Input: part model. Units: mm. Frame: model coordinates. A direction names the side the tool comes from. Round coordinates to 2 decimals unless told otherwise and drop trailing zeros. Loops run counter-clockwise (first coordinate to the right, second up) from the corner with the lowest first, then second, coordinate; pieces in that order, holes last.
1) Section C-C, the plane z = 272. Return loops of the section in (x, y), and give its area (3 significant figures).
2) First-contact query: pin 1 (5 mm diameter, centred on x = 432.5, z = 73.5, fed in from +Y); pin 2 (1.5 mm diameter, centred on y = 10, z = 263.5, fed in from -X); pin 3 (24 mm diameter, centred on x = -34, z = 3, fed in from +Y); pin 4 (12 mm diameter, centred on y = 4.5, z = 322.5, fed in from -X). Flat tips, straight axial feed; report the tip coordinate or a pass-through.
3) Access query for faces 5 (the face through (-5, 15, 0)), 6 (the face through (125, 15, 15)), 7 (the face through (-27, 45, 0)). Directions: +Z, -Z, +X, -X, +Y, -Y. A direction counts if a zero-diameter tool reaches every point of the face in a straight line with its end or side. Return the directions, or none.
4) Section A-A, the plane y = 13. Return loops of the section in (x, z), and give its area (3 significant figures).
5) Section B-B, the plane x = 766.5. Return loops of the section in (y, z).
6) Draft query along Y for faces 1 (the face through (697, 30, 240)), 2 (the face through (1285.01, 14.79, 568.91)), 3 (the face through (697, 0, 240)), 4 (the face through (-30, 30, 0)). Return one class per face: pulls with the +Y half, pulls with the -Y half, needs draft (parallel to the pull), parting line crosses it, or undercut.
7) Ray query, line 1 along Z through (x, y) = (300, 18.5); line 2 along Z through (x, y) = (-40, 40); line 3 along X through (y, z) = (-4.5, 0). Return the intervals inside material, ascending.
Autodesk Inventor part; units mm, degrees
ref_plane "Płaszczyzna konstrukcyjna1" through (0, 15, 0) normal (0, 1, 0) x (-1, 0, 0)
ref_plane "YZ Plane" through (0, 0, 0) normal (1, 0, 0) x (0, 1, 0)
ref_plane "XY Plane" through (0, 0, 0) normal (0, 0, 1) x (1, 0, 0)
sketch "Szkic1" plane through (0, 0, 0) normal (0, 1, 0) x (-1, 0, 0)
  line L0 (0, 15) -> (-300, 15)
  line L1 (-300, 15) -> (-300, -15)
  line L2 (-300, -15) -> (0, -15)
  line L3 (0, -15) -> (0, 15)
  line L4 (-300, 15) -> (-1278.6087, 580)
  line L5 (-1278.6087, 580) -> (-1291.5991, 557.5)
  line L6 (-300, -15) -> (-1291.5991, 557.5)
  point P0 (0, 0)
  point P1 (0, 0)
  dimension "d0" = 300
  dimension "d1" = 30
  dimension "d2" = 150
  dimension "d3" = 1130
extrude "Wyciągnięcie proste1" add sketch "Szkic1" along normal blind 30
sketch "Szkic2" plane through (0, 30, 0) normal (0, 1, 0) x (1, 0, 0)
  circle A0 centre (300, 0) radius 10
  line L0 (300, 15) -> (0, 15)
  point P0 (0, 0)
  dimension "d6" = 20
  dimension "d7" = 15
extrude "Wyciągnięcie proste2" cut sketch "Szkic2" against normal through all
sketch "Szkic3" plane through (0, 0, -15) normal (-1, 0, 0) x (0, 0, 1)
  point P0 (15, 0)
sketch "Szkic4" plane through (0, 0, -15) normal (-1, 0, 0) x (0, 0, 1)
  line L0 (0, 0) -> (30, 0)
  line L1 (30, 0) -> (30, 30)
  line L2 (0, 30) -> (30, 30)
  line L3 (0, 0) -> (0, 30)
  line L4 (30, 45) -> (0, 45)
  line L5 (0, 45) -> (0, -15)
  line L6 (0, -15) -> (30, -15)
  line L7 (30, -15) -> (30, 45)
  line L8 (30, 45) -> (0, -15) construction
  line L9 (0, 45) -> (30, -15) construction
  point P0 (15, 0)
  point P1 (15, 15)
  dimension "d10" = 30
  dimension "d11" = 60
  dimension "d12" = 0
  dimension "d13" = 15
extrude "Wyciągnięcie proste3" add sketch "Szkic4" along normal blind 5
sketch "Szkic5" plane through (-5, 0, -15) normal (-1, 0, 0) x (0, 0, 1)
  line L0 (0, -15) -> (30, -15)
  line L1 (30, -15) -> (30, 0)
  line L2 (30, 0) -> (0, 0)
  line L3 (0, 0) -> (0, -15)
  point P0 (15, 0)
  dimension "d16" = 30
  dimension "d17" = 15
extrude "Wyciągnięcie proste4" add sketch "Szkic5" along normal blind 50
ref_plane "Płaszczyzna konstrukcyjna1" through (0, 15, 0) normal (0, 1, 0) x (-1, 0, 0)
mirror "Odbicie lustrzane1" about plane through (0, 15, 0) normal (0, 1, 0) of "Wyciągnięcie proste4"
sketch "Szkic6" plane through (0, 45, 15) normal (0, 1, 0) x (1, 0, 0)
  circle A0 centre (-40, 15) radius 7.5
  line L0 (-55, 30) -> (-55, 0)
  line L1 (0, 0) -> (0, 30)
  point P0 (0, 15)
  point P1 (0, 15)
  dimension "d21" = 15
  dimension "d22" = 15
extrude "Wyciągnięcie proste5" cut sketch "Szkic6" against normal through all
properties part number "3" material "Złote"
Final values:
1. outline: (745.14, 0) - (797.1, 0) - (797.1, 30) - (745.14, 30) - close
1. area: 1,560 mm2
2. pin 1: stops at y = 30
2. pin 2: stops at x = 729.12
2. pin 3: stops at y = 45
2. pin 4: stops at x = 822.21
3. face 5: +Z, -Z, -X
3. face 6: +Z, -X, +Y, -Y
3. face 7: +Z, -Z, +X, -X, +Y
4. outline: (-5, -15) - (300, -15) - (1291.6, 557.5) - (1278.61, 580) - (300, 15) - (-5, 15) - close; hole circle Ø20 at (300, 0)
4. area: 38,400 mm2
5. outline: (0, 254.33) - (30, 254.33) - (30, 284.33) - (0, 284.33) - close
6. face 1: pulls with the +Y half
6. face 2: needs draft
6. face 3: pulls with the -Y half
6. face 4: undercut
7. line 1: z = -15 to -10, 10 to 15
7. line 2: z = -15 to -7.5, 7.5 to 15
7. line 3: x = -55 to -47.5, -32.5 to 0
